Autodesk Inventor part; units mm, degrees
ref_plane "YZ Plane" through (0, 0, 0) normal (1, 0, 0) x (0, 1, 0)
ref_plane "XZ Plane" through (0, 0, 0) normal (0, 1, 0) x (-1, 0, 0)
ref_plane "XY Plane" through (0, 0, 0) normal (0, 0, 1) x (1, 0, 0)
sketch "スケッチ1" plane through (0, 0, 0) normal (0, 0, 1) x (1, 0, 0)
  circle A0 centre (0, 0) radius 4.5
  circle A1 centre (0, 0) radius 6 construction
  circle A2 centre (0, 6) radius 1.1
  circle A3 centre (-4.2426, 4.2426) radius 1.1
  circle A4 centre (-6, 0) radius 1.1
  circle A5 centre (-4.2426, -4.2426) radius 1.1
  circle A6 centre (0, -6) radius 1.1
  circle A7 centre (4.2426, -4.2426) radius 1.1
  circle A8 centre (6, 0) radius 1.1
  circle A9 centre (4.2426, 4.2426) radius 1.1
  circle A10 centre (0, 0) radius 9.1
  line L0 (0, 9.1) -> (114, 9.1)
  line L1 (114, 9.1) -> (114, -9.1)
  line L2 (114, -9.1) -> (0, -9.1)
  line L3 (0, -9.1) -> (0, 9.1) construction
  line L4 (57, 9.1) -> (57, -9.1) construction
  circle A11 centre (114, 0) radius 4.5
  circle A12 centre (114, 0) radius 6 construction
  circle A13 centre (114, 6) radius 1.1
  circle A14 centre (118.2426, 4.2426) radius 1.1
  circle A15 centre (120, 0) radius 1.1
  circle A16 centre (118.2426, -4.2426) radius 1.1
  circle A17 centre (114, -6) radius 1.1
  circle A18 centre (109.7574, -4.2426) radius 1.1
  circle A19 centre (108, 0) radius 1.1
  circle A20 centre (109.7574, 4.2426) radius 1.1
  circle A21 centre (114, 0) radius 9.1
  line L5 (114, -9.1) -> (114, 9.1) construction
  point P0 (0, 0)
  point P1 (0, -9.1)
  point P2 (114, -9.1)
  dimension "d1" = 12
  dimension "d0" = 9
  dimension "d2" = 2.2
  dimension "d5" = 360
  dimension "d7" = 2
  dimension "d8" = 57
extrude "押し出し1" add sketch "スケッチ1" along normal blind 2 contours A10 | A10 L0 A21 L2 | A21 L1 A17 A11 A13 | L1 A13 A11 A17 A21
sketch "スケッチ2" plane through (0, 0, 2) normal (0, 0, 1) x (1, 0, 0)
  line L0 (52, -1.5) -> (62, -1.5)
  line L1 (62, -1.5) -> (62, 1.5)
  line L2 (62, 1.5) -> (52, 1.5)
  line L3 (52, 1.5) -> (52, -1.5)
  line L4 (114, 9.1) -> (0, 9.1)
  circle A0 centre (53.05, 1.5) radius 1.05
  line L5 (52, 0) -> (62, 0) construction
  line L6 (57, 1.5) -> (57, -1.5) construction
  circle A1 centre (60.95, 1.5) radius 1.05
  circle A2 centre (53.05, -1.5) radius 1.05
  circle A3 centre (60.95, -1.5) radius 1.05
  circle A4 centre (47, 0) radius 1.1
  circle A5 centre (67, 0) radius 1.1
  point P0 (0, 0)
  point P1 (57, 9.1)
  point P2 (59.9, 1.5)
  point P3 (54.1, 1.5)
  point P4 (54.1, -1.5)
  point P5 (59.9, -1.5)
  point P6 (62, -1.5)
  point P7 (62, 1.5)
  dimension "d13" = 2.1
  dimension "d11" = 10
  dimension "d12" = 3
  dimension "d14" = 2.2
  dimension "d15" = 5
extrude "押し出し2" cut sketch "スケッチ2" against normal blind 10
sketch "スケッチ3" plane through (0, 0, 0) normal (0, 0, -1) x (-1, 0, 0)
  line L0 (-70, -6.1) -> (-44, -6.1)
  line L1 (-44, -6.1) -> (-44, 6.1)
  line L2 (-44, 6.1) -> (-70, 6.1)
  line L3 (-70, 6.1) -> (-70, -6.1)
  line L4 (-59.9, 1.5) -> (-54.1, 1.5)
  circle A0 centre (-67, 0) radius 1.1
  line L5 (-54.1, -1.5) -> (-59.9, -1.5)
  line L6 (0, -9.1) -> (-114, -9.1)
  line L7 (-70, -6.1) -> (-114, -9.1)
  line L8 (-70, 0) -> (-120, 0) construction
  line L9 (-57, 6.1) -> (-57, 9.1) construction
  line L10 (-114, 9.1) -> (0, 9.1)
  line L11 (-70, 6.1) -> (-114, 9.1)
  line L12 (-114, -9.1) -> (0, -9.1)
  line L13 (-44, -6.1) -> (0, -9.1)
  line L14 (-44, 6.1) -> (0, 9.1)
  point P0 (0, 0)
  point P1 (-57, 1.5)
  point P2 (-57, 1.5)
  point P3 (-57, -6.1)
  point P4 (-57, -1.5)
  point P5 (0, 9.1)
  point P6 (-114, 9.1)
  dimension "d18" = 3
  dimension "d29" = 3
  dimension "d31" = 3
extrude "押し出し3" cut sketch "スケッチ3" against normal blind 10 contours L0 L13 L6 L7 | L11 L10 L14 L2
sketch "スケッチ4" plane through (0, 0, 0) normal (0, 0, -1) x (-1, 0, 0)
  line L0 (-9, 4.1405) -> (-9, -6.3815)
  line L1 (-9, -6.3815) -> (-42, -4.1315)
  line L2 (-44, -6.1) -> (0, -9.1)
  line L3 (-52, 1.5) -> (-52, -1.5)
  circle A0 centre (-6, 0) radius 1.1
  line L4 (-9, 0) -> (-26.6492, 0) construction
  circle A1 centre (-47, 0) radius 1.1 construction
  line L5 (-70, -6.1) -> (-44, -6.1) construction
  line L6 (-57, -6.1) -> (-57, 6.1) construction
  line L7 (-44, 6.1) -> (-70, 6.1) construction
  line L8 (-9, -4.1405) -> (-9, 6.3815)
  line L9 (-9, 6.3815) -> (-42, 4.1315)
  line L10 (-42, 4.1315) -> (-42, -4.1315)
  line L11 (0, 9.1) -> (-44, 6.1) construction
  line L12 (-105, 4.1405) -> (-105, -6.3815)
  line L13 (-105, -6.3815) -> (-72, -4.1315)
  line L14 (-105, 0) -> (-87.3508, 0) construction
  line L15 (-105, 6.3815) -> (-72, 4.1315)
  line L16 (-105, -4.1405) -> (-105, 6.3815)
  line L17 (-72, 4.1315) -> (-72, -4.1315)
  line L18 (-105, 6.3815) -> (-72, -4.1315)
  line L19 (-72.0515, -5.1646) -> (-105.5556, 5.509)
  line L20 (-105.5556, 5.509) -> (-104.9485, 7.4146)
  line L21 (-104.9485, 7.4146) -> (-71.4444, -3.259)
  line L22 (-71.4444, -3.259) -> (-72.0515, -5.1646)
  line L23 (-72.0515, -5.1646) -> (-104.9485, 7.4146) construction
  line L24 (-105.5556, 5.509) -> (-71.4444, -3.259) construction
  line L25 (-41.9485, -5.1646) -> (-8.4444, 5.509)
  line L26 (-9.0515, 7.4146) -> (-42.5556, -3.259)
  point P0 (0, 0)
  point P1 (-105, -4.1405)
  point P2 (-88.5, 1.125)
  point P3 (-42, -3.082)
  point P4 (-13.1915, 6.0957)
  point P5 (-9, 5.332)
  point P6 (-39.2864, -4.3165)
  point P7 (-100.8085, 6.0957)
  point P8 (-72, -3.082)
  point P9 (-74.7136, -4.3165)
  point P10 (-105, 5.332)
  dimension "d23" = 3
  dimension "d24" = 2.1
  dimension "d25" = 5
  dimension "d30" = 2
extrude "押し出し4" cut sketch "スケッチ4" against normal through all contours L0 L1 L25 L8 | L26 L10 L9 | L16 L19 L13 L12 | L15 L17 L21
fillet "フィレット1" radius 2 12 edges at (72, 4.1315, 1) (105, -6.3815, 1) (9, -6.3815, 1) (42, 4.1315, 1) (74.7136, -4.3165, 1) (72, -3.082, 1) (100.8085, 6.0957, 1) (39.2864, -4.3165, 1) (42, -3.082, 1) (13.1915, 6.0957, 1) (9, 5.332, 1) (105, 5.332, 1)
equation "\"d31\" = d29"
properties part number "腕" material "アルミニウム 2014-T4"
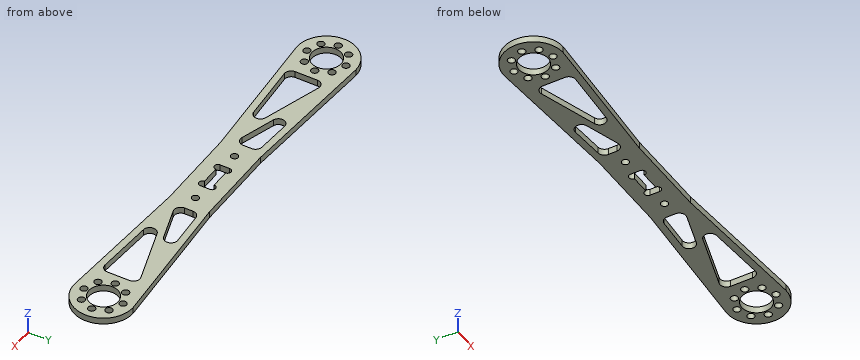
Could you check a few things on this model? Use its own coordinates, in mm. Round coordinates to 2 decimals unless told otherwise and drop trailing zeros. Write each loop counter-clockwise with the first axis right and the second up, starting at its lowest first coordinate (ties: lowest second). Pieces come first, ordered by that corner, then holes. Notation, with made-up numbers: (-21.5, 30.25) -> (-10.5, 30.25) arc R21 cw to (-10.5, 57.25) -> close; hole circle Ø11 at (58.25, -8). An arc over 180 degrees is marked (long way). Use a Markdown table: item, result.
1. If we section it at A-A (x = 67): List the corners of the cut face in (y, z) for me, then the cut area to 3 significant figures.
Answer key:
| item | result |
|---|---|
| outline | (-6.1, 0) -> (-1.1, 0) -> (-1.1, 2) -> (-6.1, 2) -> close; (1.1, 0) -> (6.1, 0) -> (6.1, 2) -> (1.1, 2) -> close |
| area | 20.0 mm^2 |
2. Please list where these lines run through material, in increasing order: probe 1 along Y at (x, z) = (114, 1.35); probe 2 along Y at (x, z) = (113, 0.8); probe 3 along Y at (x, z) = (59, 1.15).
Answer key:
| item | result |
|---|---|
| probe 1 | y = -9.1 to -7.1, -4.9 to -4.5, 4.5 to 4.9, 7.1 to 9.1 |
| probe 2 | y = -9.03 to -6.46, -5.54 to -4.39, 4.39 to 5.54, 6.46 to 9.03 |
| probe 3 | y = -6.1 to -1.5, 1.5 to 6.1 |
3. If we section it at B-B (x = 18.5): List the corners of the cut face in (y, z) for me.
Answer key:
| item | result |
|---|---|
| outline | (-7.84, 0) -> (-5.73, 0) -> (-5.73, 2) -> (-7.84, 2) -> close; (2.31, 0) -> (7.84, 0) -> (7.84, 2) -> (2.31, 2) -> close |
4. If we section it at C-C (z = 0.7): State how many separate pieces and enclosed holes the cut face has, then the cut area to 3 significant figures.
Answer key:
| item | result |
|---|---|
| separate pieces | 1 |
| enclosed holes | 25 |
| area | 1,220 mm^2 |
5. For pin 1 Ø0.6 at (x, z) = (61.5, 0.5) entering from +Y; pin 2 Ø1 at (y, z) = (-3, 1) entering from +X; pin 3 Ø0.6 at (y, z) = (1, 1.5) entering from -X, each with a flat end and sliding along its axis, tell me the tip position at first contact or that it passes through.
Answer key:
| item | result |
|---|---|
| pin 1 | stops at y = 6.1 |
| pin 2 | stops at x = 122.75 |
| pin 3 | stops at x = -9.07 |
